Read the model definition and answer for the solid it produces. Units are mm, in the model's axes. A direction names the side the tool comes from. Give positions to 0.01 mm unless a question says otherwise; leave off trailing zeros. Write each loop counter-clockwise with the first axis right and the second up, starting at its lowest first coordinate (ties: lowest second). Pieces come first, ordered by that corner, then holes. Notation, with made-up numbers: M 63,-13.5 L 89,-13.5 A21 cw 89,8.5 Z; hole C 8.5,56 d6. An arc over 180 degrees is marked long. Put each result on its own line as item: value.
from build123d import *

# Parameters (mm, degrees)
F0_W     = 38.25
F0_H     = 38.25
F1_DEPTH = 31
F0_W_2   = 95
F0_H_2   = 45
F2_DEPTH = 13
F3_R     = 6
F4_R     = 4


with BuildPart() as f1:
    # F0 (on Top) → F1 (new body)
    with BuildSketch(Plane.XY):
        with Locations((-1.875, 0.435483)):
            Rectangle(F0_W, F0_H)
    extrude(amount=F1_DEPTH)

    # F0 (on Top) → F2 (join)
    with BuildSketch(Plane.XY):
        Rectangle(F0_W_2, F0_H_2)
        with Locations((-1.875, 0.435483)):
            Rectangle(F0_W, F0_H, mode=Mode.SUBTRACT)
    extrude(amount=F2_DEPTH)

    # F3
    f3_edges = [f1.edges().sort_by_distance(p)[0] for p in [
        (-21, 19.560483, 22),
        (-21, -18.689517, 22),
        (17.25, -18.689517, 22),
        (17.25, 19.560483, 22),
    ]]
    fillet(f3_edges, radius=F3_R)

    # F4
    f4_edges = [f1.edges().sort_by_distance(p)[0] for p in [
        (47.5, -22.5, 6.5),
        (47.5, 22.5, 6.5),
        (-47.5, -22.5, 6.5),
        (-47.5, 22.5, 6.5),
    ]]
    fillet(f4_edges, radius=F4_R)


solid = f1.part
(1) Given pin 1 Ø8 at (y, z) = (-16.5, 24) entering from -X; pin 2 Ø10 at (x, z) = (-20, 19.5) entering from +Y; pin 3 Ø14.5 at (x, z) = (-5, 24.5) entering from -Y, each flat-ended and moving along its own axis, determine where each tip first touches the part or whether it passes through.
Result:
pin 1: stops at x = -21
pin 2: stops at y = 19.56
pin 3: stops at y = -18.69
(2) Section A-A on z = 22.5 is taken. Determine the outline of the cut face in (x, y), and give its area (3 significant figures).
Result:
outline: M -21,-12.69 A6 ccw -15,-18.69 L 11.25,-18.69 A6 ccw 17.25,-12.69 L 17.25,13.56 A6 ccw 11.25,19.56 L -15,19.56 A6 ccw -21,13.56 Z
area: 1,430 mm²
(3) Section C-C on x = -35 is taken. Determine the outline of the cut face in (y, z), and give its area (3 significant figures).
Result:
outline: M -22.5,0 L 22.5,0 L 22.5,13 L -22.5,13 Z
area: 585 mm²
(4) Section B-B on x = -4 is taken. Determine the outline of the cut face in (y, z), and give its area (3 significant figures).
Result:
outline: M -22.5,0 L 22.5,0 L 22.5,13 L 19.56,13 L 19.56,31 L -18.69,31 L -18.69,13 L -22.5,13 Z
area: 1,270 mm²
(5) Straight lines are drawn through the part: line 1 along Z through (x, y) = (41, -19); line 2 along X through (y, z) = (13, 13.5); line 3 along Y through (x, z) = (11.5, 22). For each, find the intervals that lie inside material, in ascending order. Write a range as from..to.
Result:
line 1: z = 0..13
line 2: x = -21..17.25
line 3: y = -18.68..19.56
(6) Which of the six approach directions +Z, -Z, +X, -X, +Y, -Y give full straight-line access (tool end or side, diameter ignored) to faces 1 (the face through (17.25, 0, 22)), 2 (the face through (15.539, 17.756, 22.126)), 3 (the face through (15.446, -16.979, 22.126)), 4 (the face through (-2, -18.69, 22))?
Result:
face 1: +Z, +X, +Y, -Y
face 2: +Z, +X, +Y
face 3: +Z, +X, -Y
face 4: +Z, +X, -X, -Y
